Part model, mm, in its own coordinate system. A direction names the side the tool comes from. Round coordinates to 2 decimals unless told otherwise and drop trailing zeros.
(1) Mould opens along X. For faces 4 (the face through (-52.25, -2, 104)), 5 (the face through (-89.14, -1.52, 124.1)), 6 (the face through (-45, -1, 125)) say: +X half, -X half, draft (parallel to the pull), parting line (faces both ways), or undercut.
(2) Cut at A-A on y = -1.4. Count the separate pieces of the cut face and the enclosed holes in it, then the cut area to 3 significant figures.
(3) Probe probe 1 along X at (y, z) = (-1.7, 66); probe 2 along X at (y, z) = (-0.55, -38); probe 3 along X at (y, z) = (-1.3, 93.5). List the from-to ranges inside material, lowest first.
(4) Tool access for faces 1 (the face through (-11, -2, 120)), 2 (the face through (-90, -1, 65)), 3 (the face through (-11, -2, 65)): list every direction of +Z, -Z, +X, -X, +Y, -Y with a clear straight run to the whole face (end or side of a thin tool).
from build123d import *

# Parameters (mm, degrees)
F0_W      = 90
F0_H      = 125
F1_DEPTH  = 3
F3_R      = 2.5
F3_R_2    = 1.5
F4_DEPTH  = 25.4
F5_R      = 25.4
F2_W      = 3
F2_H      = 5
F2_H_2    = 15
F2_H_3    = 10
F2_W_2    = 5
F2_H_4    = 3
F6_DEPTH  = 25.4
F7_W      = 3.81
F7_H      = 1.5
F7_W_2    = 1.5
F7_H_2    = 3.81
F7_R      = 1.5
F8_DEPTH  = 25.4
F9_R      = 3
F11_DEPTH = 25.4
F12_R     = 25.4
F13_R     = 1.5
F14_DEPTH = 3
F16_DEPTH = 3


# Not quite as in the source:
# - a feature names something its author has since deleted; it is built from what else it names


with BuildPart() as f1:
    # F0 (on Front) → F1 (new body)
    with BuildSketch(Plane.XZ):
        with Locations((-45, 62.5)):
            Rectangle(F0_W, F0_H)
        Polygon((-45, -70), (0, 0), (-90, 0), align=None)
    extrude(amount=F1_DEPTH)

    # F3 (on face) → F4 (cut)
    with BuildSketch(Plane.XZ.offset(3)):
        Polygon((-59, 115), (-63.75, 115), (-63.75, 109), (-58, 109), (-58, 115), align=None)
        Polygon((-58, 109), (-63.75, 109), (-63.75, 92.8), (-59, 92.8), (-58, 92.8), align=None)
        Polygon((-57, 115), (-58, 115), (-58, 109), (-52.25, 109), (-52.25, 115), align=None)
        Polygon((-52.25, 109), (-58, 109), (-58, 92.8), (-57, 92.8), (-52.25, 92.8), align=None)
        with Locations((-31, 109)):
            Circle(F3_R)
        with Locations((-17, 109)):
            Circle(F3_R_2)
    extrude(amount=-F4_DEPTH, mode=Mode.SUBTRACT)

    # F5
    f5_edges = [f1.edges().sort_by_distance(p)[0] for p in [
        (-45, -1.5, -70),
    ]]
    fillet(f5_edges, radius=F5_R)

    # F2 (on face) → F6 (cut)
    with BuildSketch(Plane.XZ.offset(3)):
        with Locations((-80.5, 127.5)):
            Rectangle(F2_W, F2_H)
        with Locations((-9.5, 127.5)):
            Rectangle(F2_W, F2_H)
        with Locations((-9.5, 65.5)):
            Rectangle(F2_W, F2_H_2)
        with Locations((-80.5, 65.5)):
            Rectangle(F2_W, F2_H_2)
        with Locations((-80.5, 120)):
            Rectangle(F2_W, F2_H_3)
        with Locations((-9.5, 120)):
            Rectangle(F2_W, F2_H_3)
        with Locations((-52.5, 56.5)):
            Rectangle(F2_W_2, F2_H_4)
        with Locations((-37.5, 56.5)):
            Rectangle(F2_W_2, F2_H_4)
    extrude(amount=-F6_DEPTH, mode=Mode.SUBTRACT)

    # F7 (on face) → F8 (cut)
    with BuildSketch(Plane.XZ.offset(3)):
        with Locations((-58.495, -22.2788609758)):
            Rectangle(F7_W, F7_H)
        with Locations((-58.495, -23.7788609758)):
            Rectangle(F7_W, F7_H)
        with Locations((-31.505, -22.2788609758)):
            Rectangle(F7_W, F7_H)
        with Locations((-31.505, -23.7788609758)):
            Rectangle(F7_W, F7_H)
        with Locations((-44.25, -36.5238609758)):
            Rectangle(F7_W_2, F7_H_2)
        with Locations((-45.75, -36.5238609758)):
            Rectangle(F7_W_2, F7_H_2)
        with Locations((-44.25, -9.5338609758)):
            Rectangle(F7_W_2, F7_H_2)
        with Locations((-45.75, -9.5338609758)):
            Rectangle(F7_W_2, F7_H_2)
        with Locations((-57.9, -9.1288609758)):
            Circle(F7_R)
        with Locations((-32.1, -10.1288609758)):
            Circle(F7_R)
        with Locations((-32.1, -35.9288609758)):
            Circle(F7_R)
        with Locations((-57.9, -35.9288609758)):
            Circle(F7_R)
    extrude(amount=-F8_DEPTH, mode=Mode.SUBTRACT)

    # F9
    f9_edges = [f1.edges().sort_by_distance(p)[0] for p in [
        (0, -1.5, 125),
        (-90, -1.5, 125),
    ]]
    fillet(f9_edges, radius=F9_R)

    # F10 (on face) → F11 (cut)
    with BuildSketch(Plane.XZ.offset(3)):
        with BuildLine():
            ThreePointArc((-66.3659332746, -36.7641037951), (-69.3706247886, -30.1865594475), (-70.4, -23.0288609758))
            Line((-70.4, -23.0288609758), (-90, 0))
            Line((-90, 0), (-66.3659332746, -36.7641037951))
        make_face()
        with BuildLine():
            Line((0, 0), (-19.6, -23.0288609758))
            ThreePointArc((-19.6, -23.0288609758), (-20.6293752114, -30.1865594475), (-23.6340667254, -36.7641037951))
            Line((-23.6340667254, -36.7641037951), (0, 0))
        make_face()
    extrude(amount=-F11_DEPTH, mode=Mode.SUBTRACT)

    # F12
    f12_edges = [f1.edges().sort_by_distance(p)[0] for p in [
        (-70.4, -1.5, -23.028861),
        (-90, -1.5, 0),
        (-19.6, -1.5, -23.028861),
        (0, -1.5, 0),
    ]]
    fillet(f12_edges, radius=F12_R)

    # F13 (on face) → F14 (cut, through all)
    with BuildSketch(Plane(origin=(0, 0, 0), x_dir=(-1, 0, 0), z_dir=(0, 1, 0))):
        with Locations((23, 61)):
            Circle(F13_R)
        with Locations((23, 35)):
            Circle(F13_R)
        with Locations((67, 35)):
            Circle(F13_R)
        with Locations((67, 61)):
            Circle(F13_R)
    extrude(amount=-F14_DEPTH, mode=Mode.SUBTRACT)

    # F15 (on face) → F16 (cut)
    with BuildSketch(Plane.XZ.offset(3)):
        with BuildLine():
            ThreePointArc((-57.2929937846, 6.804616942), (-60.2929937846, 9.804616942), (-63.2929937846, 6.804616942))
            ThreePointArc((-63.2929937846, 6.804616942), (-60.2929937846, 3.804616942), (-57.2929937846, 6.804616942))
        make_face()
    extrude(amount=-F16_DEPTH, mode=Mode.SUBTRACT)


solid = f1.part
Final values:
1. face 4: undercut
1. face 5: -X half
1. face 6: draft
2. separate pieces: 1
2. enclosed holes: 20
2. area: 13,300 mm2
3. probe 1: x = -90 to -82, -79 to -11, -8 to 0
3. probe 2: x = -65.52 to -46.5, -43.5 to -24.48
3. probe 3: x = -90 to -63.75, -52.25 to 0
4. face 1: +Z, +Y, -Y
4. face 2: +Z, -Z, -X, +Y, -Y
4. face 3: +Y, -Y
